CAD build for the part. Positions are in the model's coordinates, mm. A direction names the side the tool comes from. Coordinates: 2 decimals unless noted, no trailing zeros. Order: outer loops, then holes, each group sorted by start corner. A loop starts at its lowest first (then second) coordinate and runs counter-clockwise, first axis right, second up. Notation, with made-up numbers: M 63.25,-35 L 107.25,-35 A21 ccw 107.25,-10 Z; hole C -27.75,-38 d8. An arc over 180 degrees is marked long. Write item = value, one per line.
from build123d import *

# Parameters (mm, degrees)
SKETCH1_R             = 15
SKETCH1_R_2           = 5
BOSS_EXTRUDE1_DEPTH   = 7.5
SKETCH2_R             = 15
SKETCH2_R_2           = 7.5
BOSS_EXTRUDE2_DEPTH   = 5.5
BOSS_EXTRUDE3_START   = 5
SKETCH3_R             = 15
BOSS_EXTRUDE3_DEPTH   = 5
M4X0_7_TAPPED_HOLE1_D = 3.3
FILLET1_R             = 8
HOLE1_D               = 5
HOLE1_DEPTH           = 18
HOLE1_CBORE_D         = 7
HOLE1_CBORE_DEPTH     = 7
HOLE1_TIP             = 1.502151548
CUT_EXTRUDE1_START    = -5.5
CUT_EXTRUDE1_DEPTH    = 5.5
SKETCH10_R            = 2
BOSS_EXTRUDE4_DEPTH   = 1.5
CHAMFER1_SIZE         = 0.5


with BuildPart() as part:
    # Sketch1 → Boss-Extrude1 (new body)
    with BuildSketch(Plane(origin=(0, 0, 0), x_dir=(1, 0, 0), z_dir=(0, 1, 0))):
        with Locations(Location((0, 0, 0), (0, 0, 270))):
            Circle(SKETCH1_R)
        with Locations(Location((0, 0, 0), (0, 0, 270))):
            Circle(SKETCH1_R_2, mode=Mode.SUBTRACT)
    extrude(amount=BOSS_EXTRUDE1_DEPTH)

    # Sketch2 → Boss-Extrude2 (add)
    with BuildSketch(Plane(origin=(0, 7.5, 0), x_dir=(1, 0, 0), z_dir=(0, 1, 0))):
        with Locations(Location((0, 0, 0), (0, 0, 270))):
            Circle(SKETCH2_R)
        with Locations(Location((0, 0, 0), (0, 0, 270))):
            Circle(SKETCH2_R_2, mode=Mode.SUBTRACT)
    extrude(amount=BOSS_EXTRUDE2_DEPTH)

    # Sketch3 → Boss-Extrude3 (add)
    with BuildSketch(Plane.XZ.offset(BOSS_EXTRUDE3_START)):
        with Locations(Location((0, 0, 0), (0, 0, 270))):
            Circle(SKETCH3_R)
    extrude(amount=-BOSS_EXTRUDE3_DEPTH)

    # M4x0.7 Tapped Hole1 (through all)
    with Locations(Plane(origin=(0, -5, 0), x_dir=(-1, 0, 0), z_dir=(0, -1, 0))):
        with Locations((0, 0)):
            Hole(M4X0_7_TAPPED_HOLE1_D / 2)

    # Fillet1
    fillet1_edges = [part.edges().sort_by_distance(p)[0] for p in [
        (0, -5, 15),
    ]]
    fillet(fillet1_edges, radius=FILLET1_R)

    # Hole1
    with Locations(Plane(origin=(0, -5, 0), x_dir=(-1, 0, 0), z_dir=(0, -1, 0))):
        with Locations((0, 11.25), (-11.25, 0), (0, -11.25)):
            CounterBoreHole(HOLE1_D / 2, HOLE1_CBORE_D / 2, HOLE1_CBORE_DEPTH, depth=HOLE1_DEPTH)
            with Locations((0, 0, -(HOLE1_DEPTH + HOLE1_TIP / 2))):  # 118° drill point
                Cone(0, HOLE1_D / 2, HOLE1_TIP, mode=Mode.SUBTRACT)

    # Sketch9 → Cut-Extrude1 (cut)
    with BuildSketch(Plane(origin=(0, 13, 0), x_dir=(1, 0, 0), z_dir=(0, 1, 0)).offset(CUT_EXTRUDE1_START)):
        with BuildLine():
            Line((-5.590169944, 5), (-11.590169944, 5))
            Line((-11.590169944, 5), (-11.590169944, -5))
            Line((-11.590169944, -5), (-5.590169944, -5))
            ThreePointArc((-5.590169944, -5), (-7.5, 0), (-5.590169944, 5))
        make_face()
    extrude(amount=CUT_EXTRUDE1_DEPTH, mode=Mode.SUBTRACT)

    # Sketch10 → Boss-Extrude4 (add)
    with BuildSketch(Plane(origin=(0, 7.5, 0), x_dir=(1, 0, 0), z_dir=(0, 1, 0))):
        with Locations(Location((-8.5, 0, 0), (0, 0, 270))):
            Circle(SKETCH10_R)
    extrude(amount=BOSS_EXTRUDE4_DEPTH)

    # Chamfer1
    chamfer1_edges = [part.edges().sort_by_distance(p)[0] for p in [
        (-8.5, 9, -2),
    ]]
    chamfer(chamfer1_edges, length=CHAMFER1_SIZE)


solid = part.part
(1) Tool access for faces 4 (the face through (8.752, 7.577, -0.11)), 5 (the face through (-4.03, 7.5, 3.23)), 6 (the face through (0.46, -0.76, 7.78)): list every direction of +Z, -Z, +X, -X, +Y, -Y with a clear straight run to the whole face (end or side of a thin tool).
Evaluation:
face_4 = +Y, -Y
face_5 = +Y
face_6 = -Y
(2) Slice it at A-A, the plane y = 3.5. Write the cut outline in (x, z).
Evaluation:
outline = C 0,0 d30; hole C 0,0 d10; hole C 0,-11.25 d5; hole C 0,11.25 d5; hole C 11.25,0 d5
(3) Slice it at B-B, the plane z = 0. State how many separate pieces and enclosed holes the cut face has, then the cut area to 3 significant figures.
Evaluation:
separate_pieces = 3
enclosed_holes = 0
area = 230 mm²
(4) Wall check: line 1 (Z direction, x = 2.5, y = 0.5); line 2 (Z direction, x = 0, y = -2.5); line 3 (X direction, y = 5, z = 2). Give the ranges that are in metal, low to high. Write a range as from..to.
Evaluation:
line_1 = -14.38..-13.7, -8.8..-4.33, 4.33..8.8, 13.7..14.38
line_2 = -7.75..-1.65, 1.65..7.75
line_3 = -14.87..-4.58, 4.58..9.75, 12.75..14.87
(5) Pin check, flat tips, straight feed: pin 1 Ø1.6 at (x, y) = (-10, 9.5) entering from +Z; pin 2 Ø1.5 at (x, z) = (-8.5, -0.5) entering from +Y; pin 3 Ø4.5 at (x, z) = (0, 0) entering from +Y; pin 4 Ø3 at (x, z) = (11.25, 0) entering from -Y. Stop position of each tip, or through.
Evaluation:
pin_1 = 11.85
pin_2 = 9
pin_3 = 0
pin_4 = through
(6) Pull direction Z, two halves, no side cores. Call faces 1 (the face through (13.31, 7.93, 6.92)), 2 (the face through (-6.517, 7.993, -0.26)), 3 (the face through (7, 13, -4)): +Z half, -Z half, draft (parallel to the pull), parting line (faces both ways), or undercut.
Evaluation:
face_1 = parting line
face_2 = undercut
face_3 = draft
